The listing builds one solid part. Answer for the finished solid, in the listing's coordinates (mm). Round coordinates to 2 decimals unless told otherwise and drop trailing zeros. Order: outer loops, then holes, each group sorted by start corner. A loop starts at its lowest first (then second) coordinate and runs counter-clockwise, first axis right, second up. Notation, with made-up numbers: M 44,-35.75 L 61,-35.75 A26 cw 61,2.25 Z; hole C 68.5,44 d7. An arc over 180 degrees is marked long. Put each result on its own line as item: value. Start each with the question number.
1. The part is cut by section B-B (z = -19.5). Give the vertices of the cut face in (x, y), then the cut area to 3 significant figures.
2. The part is cut by section C-C (x = -49). Give the vertices of the cut face in (y, z).
3. Consider line 1 (Z direction, x = -33, y = -1); line 2 (X direction, y = -1.9, z = -8). Determine where each line is inside the solid, lowest interval first.
4. The part is cut by section A-A (x = -20.5). Give the vertices of the cut face in (y, z), then the cut area to 3 significant figures.
5. The part is cut by section D-D (z = 48). Give the vertices of the cut face in (x, y), then the cut area to 3 significant figures.
from build123d import *

# Parameters (mm, degrees)
F0_W     = 70
F0_H     = 70
F1_DEPTH = 3


with BuildPart() as f1:
    # F0 (on Front) → F1 (new body)
    with BuildSketch(Plane.XZ):
        Polygon((64.925, -100), (100, -100), (100, -64.925), (96.95, -64.925), (96.95, -45.025), (100, -45.025), (100, -9.95), (96.95, -9.95), (96.95, 9.95), (100, 9.95), (100, 45.025), (96.95, 45.025), (96.95, 64.925), (100, 64.925), (100, 100), (64.925, 100), (64.925, 96.95), (45.025, 96.95), (45.025, 100), (9.95, 100), (9.95, 96.95), (-9.95, 96.95), (-9.95, 100), (-45.025, 100), (-45.025, 96.95), (-64.925, 96.95), (-64.925, 100), (-100, 100), (-100, 64.925), (-96.95, 64.925), (-96.95, 45.025), (-100, 45.025), (-100, 9.95), (-96.95, 9.95), (-96.95, -9.95), (-100, -9.95), (-100, -45.025), (-96.95, -45.025), (-96.95, -64.925), (-100, -64.925), (-100, -100), (-64.925, -100), (-64.925, -96.95), (-45.025, -96.95), (-45.025, -100), (-9.95, -100), (-9.95, -96.95), (9.95, -96.95), (9.95, -100), (45.025, -100), (45.025, -96.95), (64.925, -96.95), align=None)
        Rectangle(F0_W, F0_H, mode=Mode.SUBTRACT)
    extrude(amount=F1_DEPTH)


solid = f1.part
Resolved:
1. outline: M -100,-3 L -35,-3 L -35,0 L -100,0 Z; M 35,-3 L 100,-3 L 100,0 L 35,0 Z
1. area: 390 mm2
2. outline: M -3,-96.95 L 0,-96.95 L 0,96.95 L -3,96.95 Z
3. line 1: -100 to -35, 35 to 100
3. line 2: -96.95 to -35, 35 to 96.95
4. outline: M -3,-100 L 0,-100 L 0,-35 L -3,-35 Z; M -3,35 L 0,35 L 0,100 L -3,100 Z
4. area: 390 mm2
5. outline: M -96.95,-3 L 96.95,-3 L 96.95,0 L -96.95,0 Z
5. area: 582 mm2
